```python
from build123d import *

# Parameters (mm, degrees)
EXTRUDE_1_DEPTH     = 2
SKETCH_3_W          = 2
SKETCH_3_H          = 76
EXTRUDE_2_DEPTH     = 70
SKETCH_5_R          = 28
CUT_EXTRUDE_1_DEPTH = 209.086520467
FILLET_1_R          = 0.5
FILLET_2_R          = 1.8
FILLET_3_R          = 3.8
FILLET_4_R          = 2
SKETCH_6_R          = 9
CUT_EXTRUDE_2_DEPTH = 209.086520467
CUT_EXTRUDE_3_DEPTH = 10


with BuildPart() as part:
    # Эскиз1 → Бобышка-Вытянуть1 (new body)
    with BuildSketch(Plane(origin=(0, 0, 0), x_dir=(1, 0, 0), z_dir=(0, 1, 0))):
        Polygon((52, 0), (115, 0), (120, 22), (152, 22), (152, 98), (120, 98), (115, 120), (52, 120), (47, 98), (-2, 98), (-2, 22), (47, 22), align=None)
    extrude(amount=EXTRUDE_1_DEPTH)

    # Эскиз3 → Бобышка-Вытянуть2 (add)
    with BuildSketch(Plane(origin=(0, 2, 0), x_dir=(1, 0, 0), z_dir=(0, 1, 0))):
        with Locations((-1, 60)):
            Rectangle(SKETCH_3_W, SKETCH_3_H)
        with Locations((151, 60)):
            Rectangle(SKETCH_3_W, SKETCH_3_H)
    extrude(amount=EXTRUDE_2_DEPTH)

    # Эскиз5 → Вырез-Вытянуть1 (cut, through all)
    with BuildSketch(Plane.ZY.offset(2)):
        with Locations((-60, 65.477437004)):
            Circle(SKETCH_5_R)
        Polygon((-95.299672715, 59.821425916), (-91.361232517, 59.821425916), (-91.361232517, 51.821425916), (-95.299672715, 51.821425916), (-98, 49.121098631), (-98, 72), (-90.614846418, 72), align=None)
        Polygon((-22, 72), (-22, 49.121098631), (-24.700327285, 51.821425916), (-28.638767483, 51.821425916), (-28.638767483, 59.821425916), (-24.700327285, 59.821425916), (-29.385153582, 72), align=None)
    extrude(amount=-CUT_EXTRUDE_1_DEPTH, mode=Mode.SUBTRACT)

    # Скругление1
    fillet_1_edges = [part.edges().sort_by_distance(p)[0] for p in [
        (-1, 49.121098631, -22),
        (151, 49.121098631, -22),
        (-1, 51.821425916, -24.700327285),
        (151, 51.821425916, -24.700327285),
        (-1, 51.821425916, -28.638767483),
        (151, 51.821425916, -28.638767483),
        (-1, 59.821425916, -28.638767483),
        (151, 59.821425916, -28.638767483),
        (-1, 59.821425916, -24.700327285),
        (151, 59.821425916, -24.700327285),
        (-1, 59.821425916, -95.299672715),
        (151, 59.821425916, -95.299672715),
        (-1, 59.821425916, -91.361232517),
        (151, 59.821425916, -91.361232517),
        (-1, 51.821425916, -91.361232517),
        (151, 51.821425916, -91.361232517),
        (-1, 51.821425916, -95.299672715),
        (151, 51.821425916, -95.299672715),
        (-1, 49.121098631, -98),
        (151, 49.121098631, -98),
    ]]
    fillet(fillet_1_edges, radius=FILLET_1_R)

    # Скругление2
    fillet_2_edges = [part.edges().sort_by_distance(p)[0] for p in [
        (0, 2, -60),
        (150, 2, -60),
    ]]
    fillet(fillet_2_edges, radius=FILLET_2_R)

    # Скругление3
    fillet_3_edges = [part.edges().sort_by_distance(p)[0] for p in [
        (152, 0, -60),
        (-2, 0, -60),
    ]]
    fillet(fillet_3_edges, radius=FILLET_3_R)

    # Скругление4
    fillet_4_edges = [part.edges().sort_by_distance(p)[0] for p in [
        (115, 1, -120),
        (120, 1, -98),
        (120, 1, -22),
        (115, 1, 0),
        (52, 1, 0),
        (47, 1, -22),
        (47, 1, -98),
        (52, 1, -120),
    ]]
    fillet(fillet_4_edges, radius=FILLET_4_R)

    # Эскиз6 → Вырез-Вытянуть2 (cut, through all)
    with BuildSketch(Plane.ZY.offset(2)):
        with Locations((-78.5, 22)):
            Circle(SKETCH_6_R)
        with Locations((-41.5, 22)):
            Circle(SKETCH_6_R)
    extrude(amount=-CUT_EXTRUDE_2_DEPTH, mode=Mode.SUBTRACT)

    # Эскиз7 → Вырез-Вытянуть3 (cut)
    with BuildSketch(Plane(origin=(0, 2, 0), x_dir=(1, 0, 0), z_dir=(0, 1, 0))):
        with BuildLine():
            Line((65.5, 25), (65.5, 6.5))
            ThreePointArc((65.5, 6.5), (62, 3), (58.5, 6.5))
            Line((58.5, 6.5), (58.5, 25))
            ThreePointArc((58.5, 25), (62, 28.5), (65.5, 25))
        make_face()
        with BuildLine():
            Line((108.5, 25), (108.5, 6.5))
            ThreePointArc((108.5, 6.5), (105, 3), (101.5, 6.5))
            Line((101.5, 6.5), (101.5, 25))
            ThreePointArc((101.5, 25), (105, 28.5), (108.5, 25))
        make_face()
        with BuildLine():
            Line((101.5, 95), (101.5, 113.5))
            ThreePointArc((101.5, 113.5), (105, 117), (108.5, 113.5))
            Line((108.5, 113.5), (108.5, 95))
            ThreePointArc((108.5, 95), (105, 91.5), (101.5, 95))
        make_face()
        with BuildLine():
            Line((58.5, 95), (58.5, 113.5))
            ThreePointArc((58.5, 113.5), (62, 117), (65.5, 113.5))
            Line((65.5, 113.5), (65.5, 95))
            ThreePointArc((65.5, 95), (62, 91.5), (58.5, 95))
        make_face()
    extrude(amount=-CUT_EXTRUDE_3_DEPTH, mode=Mode.SUBTRACT)


solid = part.part
```
Could you check a few things on this model? Use its own coordinates, in mm. A direction names the side the tool comes from. Give positions to 0.01 mm unless a question says otherwise; leave off trailing zeros. Write each loop counter-clockwise with the first axis right and the second up, starting at its lowest first coordinate (ties: lowest second). Pieces come first, ordered by that corner, then holes. Notation, with made-up numbers: (47.25, 1.25) -> (95.25, 1.25) arc R22 cw to (95.25, 31.25) -> close; hole circle Ø8 at (-1.75, 7.5). An arc over 180 degrees is marked (long way). Write each question's results on one line, items separated by ' | '.
1. I want a section at D-D, the plane y = 22. Write out the boundary of the cut face in (x, z), then the cut area to 3 significant figures.
Check sheet entries:
outline: (-2, -98) -> (0, -98) -> (0, -87.5) -> (-2, -87.5) -> close; (-2, -69.5) -> (0, -69.5) -> (0, -50.5) -> (-2, -50.5) -> close; (-2, -32.5) -> (0, -32.5) -> (0, -22) -> (-2, -22) -> close; (150, -98) -> (152, -98) -> (152, -87.5) -> (150, -87.5) -> close; (150, -69.5) -> (152, -69.5) -> (152, -50.5) -> (150, -50.5) -> close; (150, -32.5) -> (152, -32.5) -> (152, -22) -> (150, -22) -> close | area: 160 mm²
2. I want a section at B-B, the plane y = 6.5. Write out the boundary of the cut face in (x, z).
Check sheet entries:
outline: (-2, -98) -> (0, -98) -> (0, -22) -> (-2, -22) -> close; (150, -98) -> (152, -98) -> (152, -22) -> (150, -22) -> close
3. I want a section at A-A, the plane z = -16.5. Write out the boundary of the cut face in (x, y).
Check sheet entries:
outline: (48.25, 0) -> (58.5, 0) -> (58.5, 2) -> (48.25, 2) -> close; (65.5, 0) -> (101.5, 0) -> (101.5, 2) -> (65.5, 2) -> close; (108.5, 0) -> (118.75, 0) -> (118.75, 2) -> (108.5, 2) -> close
4. On a 3-axis mill with a long thin cutter (end or side, diameter ignored), from which of +Z, -Z, +X, -X, +Y, -Y can I reach the whole of each face in a straight line? I mean faces 1 (the flat face through (74, 2, -61)), 2 (the flat face through (150.4, 17.1, -98)), 3 (the cylindrical face through (61.9, 1, -28.5)). Say none if no direction works.
Check sheet entries:
face 1: +Z, -Z, +Y | face 2: -Z, +X, +Y, -Y | face 3: +Y, -Y
5. Will these pins go through, and if not, where does the flat tip stop? pin 1 Ø2 at (y, z) = (1.5, -19.5) entering from -X; pin 2 Ø4 at (y, z) = (58.5, -26) entering from -X; pin 3 Ø3 at (x, z) = (119, -81.5) entering from +Y; pin 4 Ø1 at (x, z) = (151.5, -93.5) entering from -Y.
Check sheet entries:
pin 1: stops at x = 47.34 | pin 2: stops at x = -2 | pin 3: stops at y = 2 | pin 4: stops at y = 1.23
6. I want a section at C-C, the plane x = 105. Write out the boundary of the cut face in (y, z).
Check sheet entries:
outline: (0, -120) -> (2, -120) -> (2, -117) -> (0, -117) -> close; (0, -91.5) -> (2, -91.5) -> (2, -28.5) -> (0, -28.5) -> close; (0, -3) -> (2, -3) -> (2, 0) -> (0, 0) -> close
7. I need wall thicknesses on L1, parallel to X at y = 44.5, z = -93; L2, parallel to Y at x = 14, z = -92.5; L3, parallel to Y at x = 151, z = -41. Which ranges of each line are inside material? Lowest first, please.
Check sheet entries:
L1: x = -2 to 0, 150 to 152 | L2: y = 0 to 2 | L3: y = 1.23 to 13.01, 30.99 to 44.91
8. If we mould it in two halves opening along Z, with no side actions, what happens to faces 4 (the cylindrical face through (150.986, 24.703, -69.916)), 5 (the flat face through (117.47, 0.99, -10.87)), 6 (the flat face through (0, 30, -59))? For each: released by +Z, released by -Z, zero draft, split by the parting line, or undercut.
Check sheet entries:
face 4: undercut | face 5: released by +Z | face 6: zero draft
